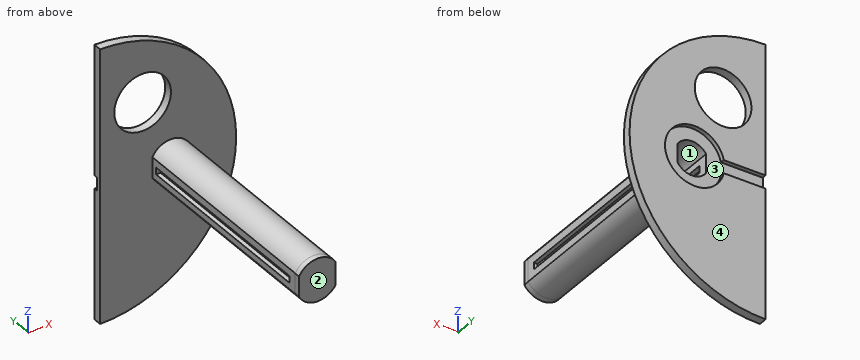
```python
from build123d import *

# Parameters (mm, degrees)
BOSS_EXTRUDE2_DEPTH = 3
CUT_EXTRUDE1_DEPTH  = 1.5
CUT_EXTRUDE4_DEPTH  = 4
BOSS_EXTRUDE4_DEPTH = 75
BOSS_EXTRUDE6_DEPTH = 2
SKETCH9_W           = 2.4
SKETCH9_H           = 70
CUT_EXTRUDE5_DEPTH  = 20
SKETCH11_R          = 10
CUT_EXTRUDE6_DEPTH  = 4


with BuildPart() as part:
    # Sketch2 → Boss-Extrude2 (new body)
    with BuildSketch(Plane(origin=(0, 0, 0), x_dir=(1, 0, 0), z_dir=(0, 1, 0))):
        with BuildLine():
            Line((0, 48), (0, -48))
            ThreePointArc((0, -48), (48, 0), (0, 48))
        make_face()
    extrude(amount=BOSS_EXTRUDE2_DEPTH)

    # Sketch3 → Cut-Extrude1 (cut)
    with BuildSketch(Plane(origin=(0, 3, 0), x_dir=(1, 0, 0), z_dir=(0, 1, 0))):
        with BuildLine():
            Line((14.75500122, 2.3), (0, 2.3))
            Line((0, 2.3), (0, -2.3))
            Line((0, -2.3), (14.75500122, -2.3))
            ThreePointArc((14.75500122, -2.3), (35.5, 0), (14.75500122, 2.3))
        make_face()
    extrude(amount=-CUT_EXTRUDE1_DEPTH, mode=Mode.SUBTRACT)

    # Sketch4 → Cut-Extrude4 (cut)
    with BuildSketch(Plane(origin=(0, 1.5, 0), x_dir=(1, 0, 0), z_dir=(0, 1, 0))):
        with BuildLine():
            Line((20, 3.31662479), (20, -3.31662479))
            ThreePointArc((20, -3.31662479), (25, -6), (30, -3.31662479))
            Line((30, -3.31662479), (30, 3.31662479))
            ThreePointArc((30, 3.31662479), (25, 6), (20, 3.31662479))
        make_face()
    extrude(amount=-CUT_EXTRUDE4_DEPTH, mode=Mode.SUBTRACT)

    # Sketch6 → Boss-Extrude4 (add)
    with BuildSketch(Plane.XZ):
        with BuildLine():
            Line((18.423549772, 3.60559321), (18.423549772, -3.60559321))
            ThreePointArc((18.423549772, -3.60559321), (24.766267094, -7.496357044), (31.339052831, -4.008292554))
            Line((31.339052831, -4.008292554), (31.339052831, 4.008292554))
            ThreePointArc((31.339052831, 4.008292554), (24.766267094, 7.496357044), (18.423549772, 3.60559321))
        make_face()
        with BuildLine():
            Line((20, 3.31662479), (20, -3.31662479))
            ThreePointArc((20, -3.31662479), (25, -6), (30, -3.31662479))
            Line((30, -3.31662479), (30, 3.31662479))
            ThreePointArc((30, 3.31662479), (25, 6), (20, 3.31662479))
        make_face(mode=Mode.SUBTRACT)
    extrude(amount=BOSS_EXTRUDE4_DEPTH)

    # Sketch8 → Boss-Extrude6 (add)
    with BuildSketch(Plane.XZ.offset(75)):
        with BuildLine():
            Line((18.4, 3.562302626), (18.4, -3.562302626))
            ThreePointArc((18.4, -3.562302626), (24.705404639, -7.494212005), (31.3, -4.06939799))
            Line((31.3, -4.06939799), (31.3, 4.06939799))
            ThreePointArc((31.3, 4.06939799), (24.705404639, 7.494212005), (18.4, 3.562302626))
        make_face()
    extrude(amount=BOSS_EXTRUDE6_DEPTH)

    # Sketch9 → Cut-Extrude5 (cut)
    with BuildSketch(Plane.ZY.offset(-18.423549772)):
        with Locations((-0.170167771, -37)):
            Rectangle(SKETCH9_W, SKETCH9_H)
    extrude(amount=-CUT_EXTRUDE5_DEPTH, mode=Mode.SUBTRACT)

    # Sketch11 → Cut-Extrude6 (cut)
    with BuildSketch(Plane(origin=(0, 3, 0), x_dir=(1, 0, 0), z_dir=(0, 1, 0))):
        with Locations((15, -24)):
            Circle(SKETCH11_R)
    extrude(amount=-CUT_EXTRUDE6_DEPTH, mode=Mode.SUBTRACT)


solid = part.part
```
Read the model definition and answer for the solid it produces. Units are mm, in the model's axes. Face numbers are marked on the shaded views. A direction names the side the tool comes from. Give positions to 0.01 mm unless a question says otherwise; leave off trailing zeros. Write each loop counter-clockwise with the first axis right and the second up, starting at its lowest first coordinate (ties: lowest second). Pieces come first, ordered by that corner, then holes. Notation, with made-up numbers: (-19.75, -25.5) -> (19.25, -25.5) arc R29 cw to (19.25, -5.5) -> close; hole circle Ø11 at (6.25, -36.75). An arc over 180 degrees is marked (long way). Answer as a JSON object with one key per item and string values.
1) Section D-D on x = 28.5 is taken. Write down the section's boundary in (y, z), then the cut area to 3 significant figures.
Findings below:
{"outline": "(-77, -6.63) -> (0, -6.63) -> (0, -38.62) -> (3, -38.62) -> (3, -9.9) -> (1.5, -9.9) -> (1.5, -4.87) -> (-75, -4.87) -> (-75, 4.87) -> (1.5, 4.87) -> (1.5, 9.9) -> (3, 9.9) -> (3, 38.62) -> (0, 38.62) -> (0, 6.63) -> (-77, 6.63) -> close", "area": "478 mm^2"}
2) Section B-B on z = 24 is taken. Write down the section's boundary in (x, y), then the cut area to 3 significant figures.
Findings below:
{"outline": "(0, 0) -> (5, 0) -> (5, 3) -> (0, 3) -> close; (25, 0) -> (41.57, 0) -> (41.57, 3) -> (25, 3) -> close", "area": "64.7 mm^2"}
3) Straight lines are drawn through the part: probe 1 along X at (y, z) = (2.75, 0); probe 2 along Y at (x, z) = (31.5, 19); probe 3 along Z at (x, y) = (28, -12.5). For each, find the intervals that lie inside material, in ascending order. Write a range as from..to.
Findings below:
{"probe 1": "x = 35.5..48", "probe 2": "y = 0..3", "probe 3": "z = -6.87..-5.2, 5.2..6.87"}
4) For a pull along X with two mould halves and no side action, classify the marked faces 3 and 4 as pulls with the +X half, pulls with the -X half, needs draft (parallel to the pull), parting line crosses it, or undercut.
Findings below:
{"face 3": "undercut", "face 4": "needs draft"}
5) Section C-C on x = 23 is taken. Write down the section's boundary in (y, z).
Findings below:
{"outline": "(-77, -7.23) -> (0, -7.23) -> (0, -42.13) -> (3, -42.13) -> (3, -10.31) -> (1.5, -10.31) -> (1.5, -5.66) -> (-75, -5.66) -> (-75, 5.66) -> (1.5, 5.66) -> (1.5, 10.31) -> (3, 10.31) -> (3, 18) -> (0, 18) -> (0, 7.23) -> (-77, 7.23) -> close; (0, 30) -> (3, 30) -> (3, 42.13) -> (0, 42.13) -> close"}
6) A tool of negligible diameter and unlimited length cuts with its end or side. For the marked faces 1 and 2, from which of +Z, -Z, +X, -X, +Y, -Y can it reach the whole face along a straight path? Write none if from no direction.
Findings below:
{"face 1": "+Y", "face 2": "+Z, -Z, +X, -X, -Y"}
7) Flat-ended cylindrical pins translate along their axes: pin 1 Ø1.1 at (x, z) = (30.5, 0) entering from +Y; pin 2 Ø6 at (x, y) = (16.5, -54.5) entering from +Z; pin 3 Ø2.5 at (y, z) = (-20, 1) entering from +X. Find the tip coordinate at first contact, or state that the pin passes through.
Findings below:
{"pin 1": "stops at y = 1.5", "pin 2": "stops at z = 5.1", "pin 3": "stops at x = 31.34"}
8) Section A-A on y = -42 is taken. Write down the section's boundary in (x, z).
Findings below:
{"outline": "(18.42, -3.61) arc R7.5 ccw to (31.34, -4.01) -> (31.34, -1.37) -> (30, -1.37) -> (30, -3.32) arc R6 cw to (20, -3.32) -> (20, -1.37) -> (18.42, -1.37) -> close; (18.42, 1.03) -> (20, 1.03) -> (20, 3.32) arc R6 cw to (30, 3.32) -> (30, 1.03) -> (31.34, 1.03) -> (31.34, 4.01) arc R7.5 ccw to (18.42, 3.61) -> close"}
